```python
from build123d import *

# Parameters (mm, degrees)
SKETCH1_W           = 61.722
SKETCH1_H           = 25.4
BOSS_EXTRUDE1_DEPTH = 6.35
SKETCH2_R           = 3.302
CUT_EXTRUDE1_DEPTH  = 7.874
CUT_EXTRUDE2_START  = -7.874
SKETCH3_R           = 3.302
CUT_EXTRUDE2_DEPTH  = 7.874
CUT_EXTRUDE11_REACH = 35.971
SKETCH4_R           = 1.75895


with BuildPart() as part:
    # Sketch1 → Boss-Extrude1 (new body)
    with BuildSketch(Plane(origin=(0, 0, 0), x_dir=(1, 0, 0), z_dir=(0, 1, 0))):
        Rectangle(SKETCH1_W, SKETCH1_H)
    extrude(amount=-BOSS_EXTRUDE1_DEPTH)

    # Sketch2 → Cut-Extrude1 (cut)
    with BuildSketch(Plane(origin=(30.861, 0, 0), x_dir=(0, 0, -1), z_dir=(1, 0, 0))):
        Circle(SKETCH2_R)
    extrude(amount=-CUT_EXTRUDE1_DEPTH, mode=Mode.SUBTRACT)

    # Sketch3 → Cut-Extrude2 (cut)
    with BuildSketch(Plane.ZY.offset(30.861).offset(CUT_EXTRUDE2_START)):
        Circle(SKETCH3_R)
    extrude(amount=CUT_EXTRUDE2_DEPTH, mode=Mode.SUBTRACT)

    # Sketch4 → Cut-Extrude11 (cut, up to next)
    with BuildSketch(Plane(origin=(0, 0, 0), x_dir=(1, 0, 0), z_dir=(0, 1, 0)), mode=Mode.PRIVATE) as cut_extrude11_sk1:
        with Locations(Location((25.30475, -8.001, 0), (0, 0, 270))):
            Circle(SKETCH4_R)
    cut_extrude11_tool1 = extrude(cut_extrude11_sk1.sketch, amount=-CUT_EXTRUDE11_REACH, mode=Mode.PRIVATE) & part.part
    # Sketch4 → Cut-Extrude11 (cut, up to next)
    with BuildSketch(Plane(origin=(0, 0, 0), x_dir=(1, 0, 0), z_dir=(0, 1, 0)), mode=Mode.PRIVATE) as cut_extrude11_sk2:
        with Locations(Location((25.30475, 8.001, 0), (0, 0, 270))):
            Circle(SKETCH4_R)
    cut_extrude11_tool2 = extrude(cut_extrude11_sk2.sketch, amount=-CUT_EXTRUDE11_REACH, mode=Mode.PRIVATE) & part.part
    # Sketch4 → Cut-Extrude11 (cut, up to next)
    with BuildSketch(Plane(origin=(0, 0, 0), x_dir=(1, 0, 0), z_dir=(0, 1, 0)), mode=Mode.PRIVATE) as cut_extrude11_sk3:
        with Locations(Location((-25.30475, 8.001, 0), (0, 0, 270))):
            Circle(SKETCH4_R)
    cut_extrude11_tool3 = extrude(cut_extrude11_sk3.sketch, amount=-CUT_EXTRUDE11_REACH, mode=Mode.PRIVATE) & part.part
    # Sketch4 → Cut-Extrude11 (cut, up to next)
    with BuildSketch(Plane(origin=(0, 0, 0), x_dir=(1, 0, 0), z_dir=(0, 1, 0)), mode=Mode.PRIVATE) as cut_extrude11_sk4:
        with Locations(Location((-25.30475, -8.001, 0), (0, 0, 270))):
            Circle(SKETCH4_R)
    cut_extrude11_tool4 = extrude(cut_extrude11_sk4.sketch, amount=-CUT_EXTRUDE11_REACH, mode=Mode.PRIVATE) & part.part
    add(cut_extrude11_tool1.solids().sort_by_distance((25.30475, 0, 8.001))[0], mode=Mode.SUBTRACT)
    add(cut_extrude11_tool2.solids().sort_by_distance((25.30475, 0, -8.001))[0], mode=Mode.SUBTRACT)
    add(cut_extrude11_tool3.solids().sort_by_distance((-25.30475, 0, -8.001))[0], mode=Mode.SUBTRACT)
    add(cut_extrude11_tool4.solids().sort_by_distance((-25.30475, 0, 8.001))[0], mode=Mode.SUBTRACT)


solid = part.part
```
Can you work these out from the model? Positions are in its coordinate system, mm. A direction names the side the tool comes from. Give positions to 0.01 mm unless a question says otherwise; leave off trailing zeros. Write each loop counter-clockwise with the first axis right and the second up, starting at its lowest first coordinate (ties: lowest second). Pieces come first, ordered by that corner, then holes. Notation, with made-up numbers: (60.5, -13) -> (71.5, -13) arc R22 cw to (71.5, 24) -> close; hole circle Ø7 at (-22.75, -35). An arc over 180 degrees is marked (long way). One line per item, written item: value.
Q1. Imagine slicing it at C-C on y = -2.75. Please give me the cut outline in (x, z).
Results found:
outline: (-30.86, -12.7) -> (30.86, -12.7) -> (30.86, -1.83) -> (22.99, -1.83) -> (22.99, 1.83) -> (30.86, 1.83) -> (30.86, 12.7) -> (-30.86, 12.7) -> (-30.86, 1.83) -> (-22.99, 1.83) -> (-22.99, -1.83) -> (-30.86, -1.83) -> close; hole circle Ø3.52 at (-25.3, -8); hole circle Ø3.52 at (-25.3, 8); hole circle Ø3.52 at (25.3, -8); hole circle Ø3.52 at (25.3, 8)
Q2. We'd pull the mould along Z, two halves only. Please class faces 1 (the face through (0, -3, 12.7)), 2 (the face through (23.588, -3.131, 7.62)), 3 (the face through (0, -6.35, 0)): +Z half, -Z half, draft (parallel to the pull), parting line (faces both ways), or undercut.
Results found:
face 1: +Z half
face 2: undercut
face 3: draft
Q3. For P1, Ø3, axis at x = 25.3, z = -8, coming from the -Y side; P2, Ø1, axis at y = -2, z = 1, coming from the -X side, each with a flat end and sliding along its axis, tell me the tip position at first contact or that it passes through.
Results found:
P1: passes through
P2: stops at x = -22.99
Q4. Imagine slicing it at A-A on z = -8. Please give me the cut outline in (x, y), and give its area (3 significant figures).
Results found:
outline: (-30.86, -6.35) -> (-27.06, -6.35) -> (-27.06, 0) -> (-30.86, 0) -> close; (-23.55, -6.35) -> (23.55, -6.35) -> (23.55, 0) -> (-23.55, 0) -> close; (27.06, -6.35) -> (30.86, -6.35) -> (30.86, 0) -> (27.06, 0) -> close
area: 347 mm^2
Q5. Imagine slicing it at D-D on z = 7.75. Please give me the cut outline in (x, y), and give its area (3 significant figures).
Results found:
outline: (-30.86, -6.35) -> (-27.05, -6.35) -> (-27.05, 0) -> (-30.86, 0) -> close; (-23.56, -6.35) -> (23.56, -6.35) -> (23.56, 0) -> (-23.56, 0) -> close; (27.05, -6.35) -> (30.86, -6.35) -> (30.86, 0) -> (27.05, 0) -> close
area: 348 mm^2
Q6. Please list where these lines run through material, in increasing order: line 1 (Z direction, x = -25.5, y = -5.25); line 2 (X direction, y = -5, z = 8); line 3 (X direction, y = -1.5, z = 7.25). Write a range as [from, to].
Results found:
line 1: z = [-12.7, -9.75], [-6.25, 6.25], [9.75, 12.7]
line 2: x = [-30.86, -27.06], [-23.55, 23.55], [27.06, 30.86]
line 3: x = [-30.86, -26.9], [-23.71, 23.71], [26.9, 30.86]
Q7. Imagine slicing it at B-B on z = 0. Please give me the cut outline in (x, y).
Results found:
outline: (-30.86, -6.35) -> (30.86, -6.35) -> (30.86, -3.3) -> (22.99, -3.3) -> (22.99, 0) -> (-22.99, 0) -> (-22.99, -3.3) -> (-30.86, -3.3) -> close
Q8. Which directions (+Z, -Z, +X, -X, +Y, -Y) give clear straight access to the entire face, cutting with the end or side of a thin tool? Please do faces 4 (the face through (-22.987, -1, 0)), 5 (the face through (22.987, -1, 0)), 6 (the face through (0, -3, -12.7)).
Results found:
face 4: -X, +Y
face 5: +X, +Y
face 6: -Z, +X, -X, +Y, -Y
